Input: dimensioned drawing with shaded views. Units: mm. Origin: part minimum x, y, z. A direction names the side the tool comes from. Round coordinates to 2 decimals unless told otherwise and drop trailing zeros. Order: outer loops, then holes, each group sorted by start corner. A loop starts at its lowest first (then second) coordinate and runs counter-clockwise, first axis right, second up.
Item 1: Cut plane B-B on y = 38.5. Output: boundary loops of the cut face in (x, z).
Item 2: Cut plane C-C on y = 25. Output: boundary loops of the cut face in (x, z) (1 decimal), then the cut area to 3 significant figures.
Item 3: Reachability of the marked faces 1 and 2 from +Z, -Z, +X, -X, +Y, -Y: full face, straight path, thin tool, end or side. Return the list, or none.
Item 4: First-contact query: pin 1 (6 mm diameter, centred on x = 3.5, y = 39.5, fed in from -Z); pin 2 (4 mm diameter, centred on y = 41.5, z = 3, fed in from -X); pin 3 (5 mm diameter, centred on x = 3, y = 36, fed in from -Z) (1 decimal). Flat tips, straight axial feed; report the tip coordinate or a pass-through.
Item 5: Line query: L1, parallel to Y at x = 10.5, z = 4; L2, parallel to Y at x = 9.75, z = 4.5; L3, parallel to Z at x = 6.25, y = 40.5. Output: solid intervals per line, ascending.
Item 6: Mould query, pull axis X, two halves, no side actions, for the marked faces 3, 4 and 5. Classes: released by +X, released by -X, zero draft, split by the parting line, or undercut.
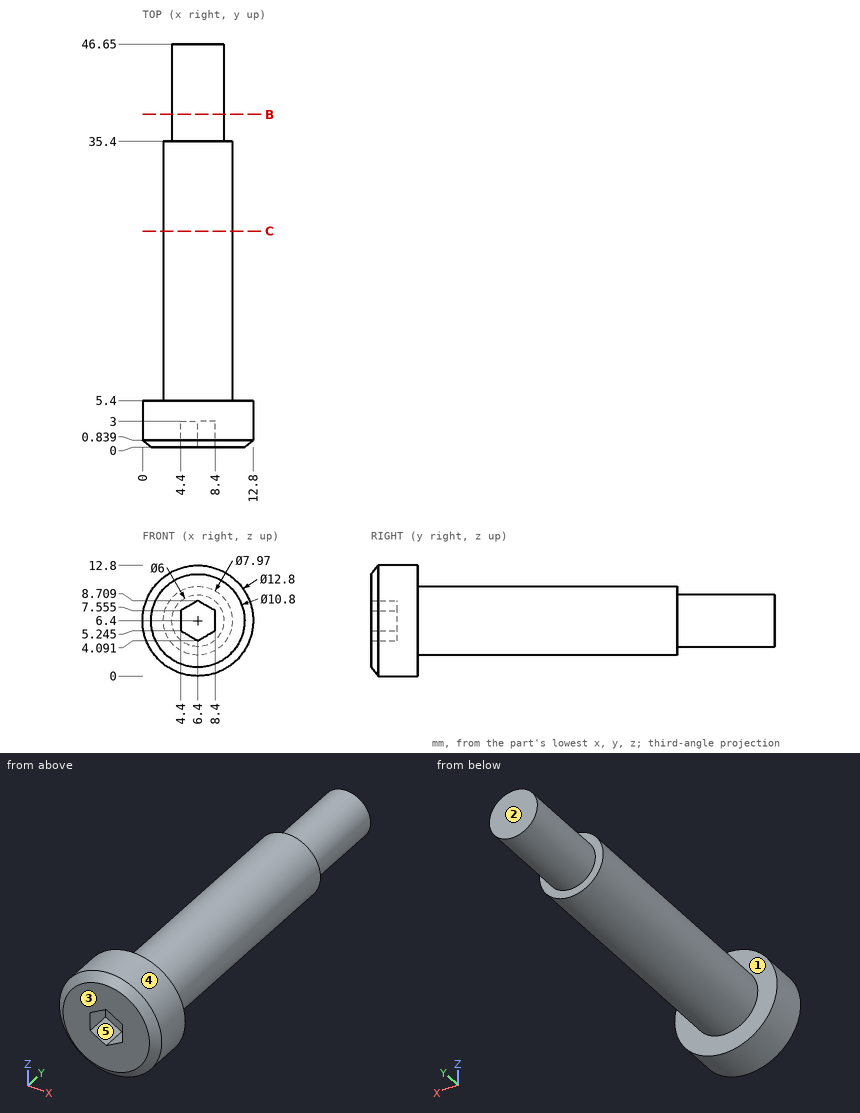
From the geometry:
1. outline: circle Ø6 at (6.4, 6.4)
2. outline: circle Ø8 at (6.4, 6.4)
2. area: 49.9 mm2
3. face 1: +Y
3. face 2: +Z, -Z, +X, -X, +Y
4. pin 1: stops at z = 3.4
4. pin 2: stops at x = 3.75
4. pin 3: stops at z = 2.5
5. L1: y = 0 to 5.4
5. L2: y = 0 to 35.4
5. L3: z = 3.4 to 9.4
6. face 3: zero draft
6. face 4: split by the parting line
6. face 5: undercut
